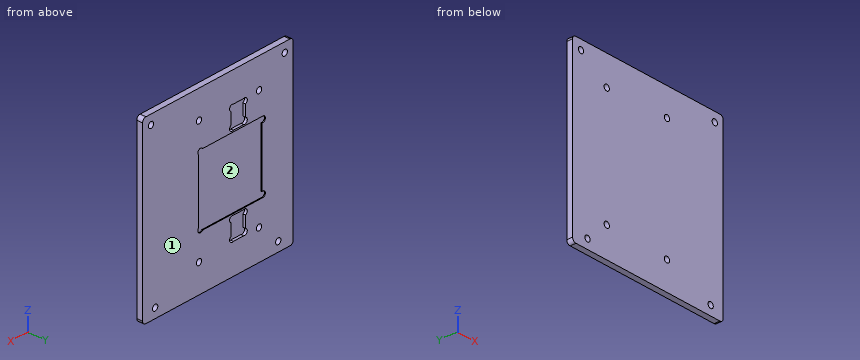
```python
from build123d import *

# Parameters (mm, degrees)
BOSS_EXTRUDE1_DEPTH = 3.175
SKETCH2_R           = 1.5875
SKETCH2_R_2         = 1.59
CUT_EXTRUDE1_DEPTH  = 132.664731895
CUT_EXTRUDE2_DEPTH  = 0.5
CUT_EXTRUDE3_DEPTH  = 1.5


with BuildPart() as part:
    # Sketch1 → Boss-Extrude1 (new body)
    with BuildSketch(Plane(origin=(0, 0, 0), x_dir=(1, 0, 0), z_dir=(0, 1, 0))):
        with BuildLine():
            Line((2, 0), (88.17, 0))
            ThreePointArc((88.17, 0), (89.584213562, 0.585786438), (90.17, 2))
            Line((90.17, 2), (90.17, 93.89))
            ThreePointArc((90.17, 93.89), (89.584213562, 95.304213562), (88.17, 95.89))
            Line((88.17, 95.89), (2, 95.89))
            ThreePointArc((2, 95.89), (0.585786438, 95.304213562), (0, 93.89))
            Line((0, 93.89), (0, 2))
            ThreePointArc((0, 2), (0.585786438, 0.585786438), (2, 0))
        make_face()
    extrude(amount=BOSS_EXTRUDE1_DEPTH)

    # Sketch2 → Cut-Extrude1 (cut, through all)
    with BuildSketch(Plane(origin=(0, 3.175, 0), x_dir=(1, 0, 0), z_dir=(0, 1, 0))):
        with Locations(Location((5.08, 5.08, 0), (0, 0, 270))):
            Circle(SKETCH2_R)
        with Locations(Location((8.96488723, 90.81, 0), (0, 0, 270))):
            Circle(SKETCH2_R)
        with Locations(Location((85.09, 5.08, 0), (0, 0, 270))):
            Circle(SKETCH2_R)
        with Locations(Location((82.62488723, 90.81, 0), (0, 0, 270))):
            Circle(SKETCH2_R)
        with Locations(Location((20.45, 16.036, 0), (0, 0, 270))):
            Circle(SKETCH2_R_2)
        with Locations(Location((20.45, 79.636, 0), (0, 0, 270))):
            Circle(SKETCH2_R)
        with Locations(Location((56.45, 80.636, 0), (0, 0, 270))):
            Circle(SKETCH2_R)
        with Locations(Location((56.45, 15.036, 0), (0, 0, 270))):
            Circle(SKETCH2_R)
    extrude(amount=-CUT_EXTRUDE1_DEPTH, mode=Mode.SUBTRACT)

    # Sketch3 → Cut-Extrude2 (cut)
    with BuildSketch(Plane(origin=(0, 3.175, 0), x_dir=(1, 0, 0), z_dir=(0, 1, 0))):
        with BuildLine():
            Line((17.786991297, 66.746), (54.196641075, 66.746))
            ThreePointArc((54.196641075, 66.746), (56.404844266, 67.151155734), (56.81, 64.942952544))
            Line((56.81, 64.942952544), (56.81, 30.729047456))
            ThreePointArc((56.81, 30.729047456), (56.404844266, 28.520844266), (54.196641075, 28.926))
            Line((54.196641075, 28.926), (17.786991297, 28.926))
            ThreePointArc((17.786991297, 28.926), (16.775636345, 30.930363655), (18.78, 31.941718607))
            Line((18.78, 31.941718607), (18.78, 63.730281393))
            ThreePointArc((18.78, 63.730281393), (16.775636345, 64.741636345), (17.786991297, 66.746))
        make_face()
    extrude(amount=-CUT_EXTRUDE2_DEPTH, mode=Mode.SUBTRACT)

    # Sketch4 → Cut-Extrude3 (cut)
    with BuildSketch(Plane(origin=(0, 3.175, 0), x_dir=(1, 0, 0), z_dir=(0, 1, 0))):
        with BuildLine():
            Line((29.63877923, 28.126), (35.86122077, 28.126))
            ThreePointArc((35.86122077, 28.126), (37.961961131, 27.334038869), (37.17, 25.233298507))
            Line((37.17, 25.233298507), (37.17, 18.898701493))
            ThreePointArc((37.17, 18.898701493), (37.961961131, 16.797961131), (35.86122077, 16.006))
            Line((35.86122077, 16.006), (29.63877923, 16.006))
            ThreePointArc((29.63877923, 16.006), (27.603149796, 16.952850204), (28.55, 18.988479638))
            Line((28.55, 18.988479638), (28.55, 25.143520362))
            ThreePointArc((28.55, 25.143520362), (27.603149796, 27.179149796), (29.63877923, 28.126))
        make_face()
        with BuildLine():
            Line((37.17, 76.753298507), (37.17, 70.418701493))
            ThreePointArc((37.17, 70.418701493), (37.961961131, 68.317961131), (35.86122077, 67.526))
            Line((35.86122077, 67.526), (29.63877923, 67.526))
            ThreePointArc((29.63877923, 67.526), (27.603149796, 68.472850204), (28.55, 70.508479638))
            Line((28.55, 70.508479638), (28.55, 76.663520362))
            ThreePointArc((28.55, 76.663520362), (27.603149796, 78.699149796), (29.63877923, 79.646))
            Line((29.63877923, 79.646), (35.86122077, 79.646))
            ThreePointArc((35.86122077, 79.646), (37.961961131, 78.854038869), (37.17, 76.753298507))
        make_face()
    extrude(amount=-CUT_EXTRUDE3_DEPTH, mode=Mode.SUBTRACT)


solid = part.part
```
CAD build for the part. Positions are in the model's coordinates, mm. Face numbers are marked on the shaded views. Give positions to 0.01 mm unless a question says otherwise; leave off trailing zeros. Order: outer loops, then holes, each group sorted by start corner. A loop starts at its lowest first (then second) coordinate and runs counter-clockwise, first axis right, second up.
(1) Drill centre lines: L1, parallel to X at y = 2.3, z = -90.81; L2, parallel to X at y = 0.9, z = -5.08; L3, parallel to Z at x = 32, y = 2.1. Where is each one in solid material? Low to high.
(2) Saw through at C-C, the plane z = -42.5. Give the cut face in (x, y) (3 decimals).
(3) Saw through at D-D, the plane x = 42. Give the cut face in (y, z) (3 decimals), then the cut area to 3 significant figures.
(4) Flat gauge pin, fed straight in: pin 1 (3 mm diameter, centred on x = 5.08, z = -5.08, fed in from -Y). Where does the tip first touch, or does it go through?
(5) Saw through at B-B, the plane z = -90.81. Give the cut face in (x, y) (3 decimals), then the cut area to 3 significant figures.
(6) Mould opens along X. For the marked faces 1 and 2 say: released by +X, released by -X, zero draft, split by the parting line, or undercut.
(7) Saw through at A-A, the plane x = 20.45. Give the cut face in (y, z) (1 decimal), then the cut area to 3 significant figures.
Results found:
1. L1: x = 0 to 7.38, 10.55 to 81.04, 84.21 to 90.17
1. L2: x = 0 to 3.49, 6.67 to 83.5, 86.68 to 90.17
1. L3: z = -95.89 to -79.65, -67.53 to -28.13, -16.01 to 0
2. outline: (0, 0) - (90.17, 0) - (90.17, 3.175) - (56.81, 3.175) - (56.81, 2.675) - (18.78, 2.675) - (18.78, 3.175) - (0, 3.175) - close
3. outline: (0, -95.89) - (3.175, -95.89) - (3.175, -66.746) - (2.675, -66.746) - (2.675, -28.926) - (3.175, -28.926) - (3.175, 0) - (0, 0) - close
3. area: 286 mm2
4. pin 1: passes through
5. outline: (0, 0) - (7.377, 0) - (7.377, 3.175) - (0, 3.175) - close; (10.552, 0) - (81.037, 0) - (81.037, 3.175) - (10.552, 3.175) - close; (84.212, 0) - (90.17, 0) - (90.17, 3.175) - (84.212, 3.175) - close
5. area: 266 mm2
6. face 1: zero draft
6. face 2: undercut
7. outline: (0, -95.9) - (3.2, -95.9) - (3.2, -81.2) - (0, -81.2) - close; (0, -78) - (3.2, -78) - (3.2, -66.7) - (2.7, -66.7) - (2.7, -28.9) - (3.2, -28.9) - (3.2, -17.6) - (0, -17.6) - close; (0, -14.4) - (3.2, -14.4) - (3.2, 0) - (0, 0) - close
7. area: 265 mm2
